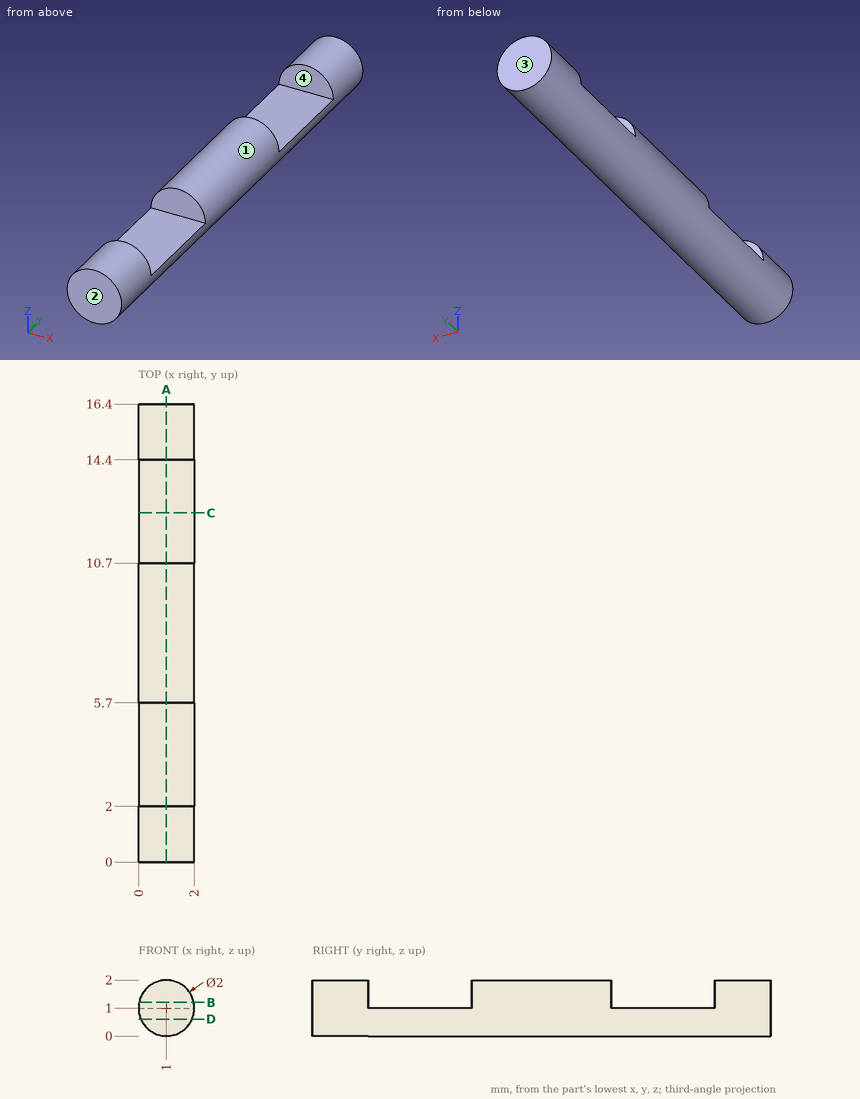
Answer from the drawing. Dimensions are ordinates in mm from the lowest x, y and z of the part. Give positions to 0.01 mm unless a question says otherwise; leave off trailing zeros. Write each loop counter-clockwise with the first axis right and the second up, starting at its lowest first coordinate (ties: lowest second). Pieces come first, ordered by that corner, then holes.
1) Given P1, Ø0.8, axis at x = 1, z = 1.5, coming from the -Y side; P2, Ø0.6, axis at x = 1, y = 13, coming from the +Z side, each flat-ended and moving along its own axis, determine where each tip first touches the part or whether it passes through.
2) Section A-A (x = 1) is taken. Write down the section's boundary in (y, z), and give its area (3 significant figures).
3) Find the intervals of material crossed by L1, parallel to Y at x = 0.65, z = 1.8; L2, parallel to X at y = 9.75, z = 0.95; L3, parallel to X at y = 8, z = 0.1, in increasing order.
4) Section C-C (y = 12.5) is taken. Write down the section's boundary in (x, z).
5) For a pull along Y with two mould halves and no side action, classify the marked faces 1, 2, 3 and 4 as pulls with the +Y half, pulls with the -Y half, needs draft (parallel to the pull), parting line crosses it, or undercut.
6) Section B-B (z = 1.2) is taken. Write down the section's boundary in (x, y), and give its area (3 significant figures).
7) Section D-D (z = 0.6) is taken. Write down the section's boundary in (x, y), and give its area (3 significant figures).
Response:
1. P1: stops at y = 0
1. P2: stops at z = 1
2. outline: (0, 0) - (16.4, 0) - (16.4, 2) - (14.4, 2) - (14.4, 1) - (10.7, 1) - (10.7, 2) - (5.7, 2) - (5.7, 1) - (2, 1) - (2, 2) - (0, 2) - close
2. area: 25.4 mm2
3. L1: y = 0 to 2, 5.7 to 10.7, 14.4 to 16.4
3. L2: x = 0 to 2
3. L3: x = 0.56 to 1.44
4. outline: (0, 1) arc R1 ccw to (2, 1) - close
5. face 1: needs draft
5. face 2: pulls with the -Y half
5. face 3: pulls with the +Y half
5. face 4: undercut
6. outline: (0.02, 0) - (1.98, 0) - (1.98, 2) - (0.02, 2) - close; (0.02, 5.7) - (1.98, 5.7) - (1.98, 10.7) - (0.02, 10.7) - close; (0.02, 14.4) - (1.98, 14.4) - (1.98, 16.4) - (0.02, 16.4) - close
6. area: 17.6 mm2
7. outline: (0.08, 0) - (1.92, 0) - (1.92, 16.4) - (0.08, 16.4) - close
7. area: 30.1 mm2
